Drawing for the job (mm, zero at the part's lowest x, y, z). A direction names the side the tool comes from. Give positions to 0.01 mm unless a question says otherwise; leave off trailing zeros. Order: outer loops, then holes, each group sorted by start corner. A loop starts at its lowest first (then second) coordinate and runs counter-clockwise, first axis right, second up. Notation, with made-up numbers: (30.5, -0.75) - (39.5, -0.75) arc R26 ccw to (39.5, 30.25) - close; hole circle Ø7 at (-21.75, -24). An arc over 180 degrees is marked (long way). One line per item, written item: value.
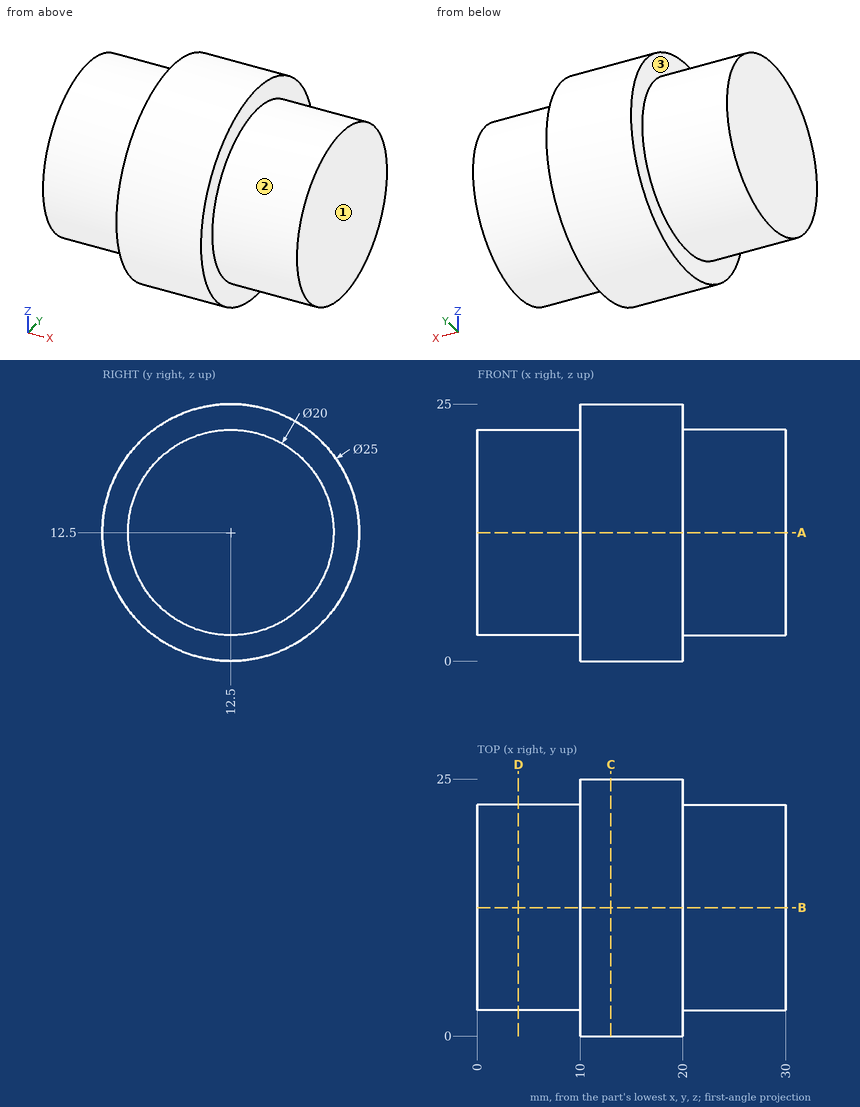
1) Which spindle directions (+Z, -Z, +X, -X, +Y, -Y) get a long thin tool onto all of the face, cutting with end or side? Do the marked faces 1, 2 and 3. Say none if no direction does.
Outcome:
face 1: +Z, -Z, +X, +Y, -Y
face 2: +X
face 3: -X
2) Drill centre lines: line 1 along Y through (x, z) = (19.25, 20); line 2 along X through (y, z) = (13.5, 1.75); line 3 along Z through (x, y) = (16.75, 12.75). Where is each one in solid material? Low to high. Write a range as from..to.
Outcome:
line 1: y = 2.5..22.5
line 2: x = 10..20
line 3: z = 0..25
3) Cut at D-D, the plane x = 4. Give the cut face in (y, z).
Outcome:
outline: circle Ø20 at (12.5, 12.5)
4) Cut at C-C, the plane x = 13. Give the cut face in (y, z), then the cut area to 3 significant figures.
Outcome:
outline: circle Ø25 at (12.5, 12.5)
area: 491 mm^2
5) Cut at A-A, the plane z = 12.5. Give the cut face in (x, y).
Outcome:
outline: (0, 2.5) - (10, 2.5) - (10, 0) - (20, 0) - (20, 2.5) - (30, 2.5) - (30, 22.5) - (20, 22.5) - (20, 25) - (10, 25) - (10, 22.5) - (0, 22.5) - close
6) Pin check, flat tips, straight feed: pin 1 (10 mm diameter, centred on x = 13, z = 18.5, fed in from +Y); pin 2 (3 mm diameter, centred on x = 23, z = 4.5, fed in from -Y); pin 3 (3 mm diameter, centred on x = 19, y = 8, fed in from -Z). Stop position of each tip, or through.
Outcome:
pin 1: stops at y = 24.96
pin 2: stops at y = 4.9
pin 3: stops at z = 0.37
